from build123d import *

# Parameters (mm, degrees)
BOSS_EXTRUDE1_DEPTH      = 8.5
CUT_EXTRUDE4_DEPTH       = 12
FILLET1_R                = 3
CUT_EXTRUDE5_DEPTH       = 46.354741112
CUT_EXTRUDE5_DEPTH_BACK  = 46.354741112
SKETCH6_W                = 4.541260622
SKETCH6_H                = 2
CUT_EXTRUDE6_START       = 1
CUT_EXTRUDE6_DEPTH       = 3
CUT_EXTRUDE7_REACH       = 47.355
CUT_EXTRUDE7_END_RADIUS  = 42.2
SKETCH8_W                = 25
SKETCH8_H                = 3
BOSS_EXTRUDE2_START      = 6.5
BOSS_EXTRUDE2_DEPTH      = 3
FILLET2_R                = 5
SKETCH10_R               = 11
CUT_EXTRUDE8_DEPTH       = 2
CUT_EXTRUDE9_REACH       = 63.124
SKETCH11_R               = 3.75
FILLET3_R                = 7.5
CUT_EXTRUDE10_DEPTH      = 61.534679882
CUT_EXTRUDE10_DEPTH_BACK = 61.534679882
SKETCH12_W               = 19.340558592
SKETCH12_H               = 3


# Read off the part's stored shape, not the designer's step: Cut-Extrude6
with BuildPart() as part:
    # Sketch1 → Boss-Extrude1 (new, symmetric)
    with BuildSketch(Plane(origin=(0, 0, 0), x_dir=(1, 0, 0), z_dir=(0, 1, 0))):
        with BuildLine():
            Line((-39.278701549, 15), (39.278701549, 15))
            ThreePointArc((39.278701549, 15), (41.95, 0), (39.278701549, -15))
            Line((39.278701549, -15), (-39.278701549, -15))
            ThreePointArc((-39.278701549, -15), (-41.95, 0), (-39.278701549, 15))
        make_face()
    extrude(amount=BOSS_EXTRUDE1_DEPTH, both=True)

    # Sketch5 → Cut-Extrude4 (cut)
    with BuildSketch(Plane(origin=(0, 8.5, 0), x_dir=(1, 0, 0), z_dir=(0, 1, 0))):
        with BuildLine():
            Line((-37.408739378, 15), (34.445827296, 15))
            ThreePointArc((34.445827296, 15), (37.45, 0), (34.445827296, -15))
            Line((34.445827296, -15), (-37.408739378, -15))
            ThreePointArc((-37.408739378, -15), (-40.2, 0), (-37.408739378, 15))
        make_face()
    extrude(amount=-CUT_EXTRUDE4_DEPTH, mode=Mode.SUBTRACT)

    # Fillet1
    fillet1_edges = [part.edges().sort_by_distance(p)[0] for p in [
        (-40.2, -3.5, 0),
        (37.45, -3.5, 0),
        (-41.95, -8.5, 0),
        (41.95, -8.5, 0),
    ]]
    fillet(fillet1_edges, radius=FILLET1_R)

    # Sketch6 → Cut-Extrude5 (cut, two sides: drawn at the far end of the back side and taken through both)
    with BuildSketch(Plane.XY.offset(-CUT_EXTRUDE5_DEPTH_BACK)):
        with Locations((-39.679369689, 7.5)):
            Rectangle(SKETCH6_W, SKETCH6_H)
    extrude(amount=CUT_EXTRUDE5_DEPTH + CUT_EXTRUDE5_DEPTH_BACK, mode=Mode.SUBTRACT)

    # Cut-Extrude6 outline → Cut-Extrude6 (cut)
    with BuildSketch(Plane(origin=(0, 0, 0), x_dir=(1, 0, 0), z_dir=(0, 1, 0)).offset(CUT_EXTRUDE6_START)):
        with BuildLine():
            ThreePointArc((-40.987968885, -4.25), (-40.485797555, -7.777069093), (-39.691352248, -11.25))
            Line((-39.691352248, -11.25), (-38.653798077, -11.25))
            ThreePointArc((-38.653798077, -11.25), (-39.468108328, -7.778438147), (-39.982857905, -4.25))
            Line((-39.982857905, -4.25), (-40.987968885, -4.25))
        make_face()
        with BuildLine():
            Line((-40.987968885, 4.25), (-39.982857905, 4.25))
            ThreePointArc((-39.982857905, 4.25), (-39.468108328, 7.778438147), (-38.653798077, 11.25))
            Line((-38.653798077, 11.25), (-39.691352248, 11.25))
            ThreePointArc((-39.691352248, 11.25), (-40.485797555, 7.777069093), (-40.987968885, 4.25))
        make_face()
    extrude(amount=CUT_EXTRUDE6_DEPTH, mode=Mode.SUBTRACT)

    # Cut-Extrude7: up to this cylinder (the profile starts inside it)
    cut_extrude7_end = Plane(origin=(-1.5, 0.5, 0), z_dir=(0, -1, 0)) * Cylinder(CUT_EXTRUDE7_END_RADIUS, 180.11, mode=Mode.PRIVATE)
    # Sketch8 → Cut-Extrude7 (cut, up to the surface)
    with BuildSketch(Plane(origin=(0, 0, 0), x_dir=(0, 0, -1), z_dir=(1, 0, 0)), mode=Mode.PRIVATE) as cut_extrude7_sk1:
        with Locations((0, 0.5)):
            Rectangle(SKETCH8_W, SKETCH8_H)
    cut_extrude7_tool1 = extrude(cut_extrude7_sk1.sketch, amount=CUT_EXTRUDE7_REACH, mode=Mode.PRIVATE) & cut_extrude7_end
    add(cut_extrude7_tool1.solids().sort_by_distance((0, 0.5, 0))[0], mode=Mode.SUBTRACT)

    # Sketch9 → Boss-Extrude2 (add)
    with BuildSketch(Plane(origin=(0, 0, 0), x_dir=(1, 0, 0), z_dir=(0, 1, 0)).offset(BOSS_EXTRUDE2_START)):
        with BuildLine():
            Line((-53.356504155, 20.178365938), (-39.278701549, 15))
            ThreePointArc((-39.278701549, 15), (-41.95, 0), (-39.278701549, -15))
            Line((-39.278701549, -15), (-53.356504155, -20.178365938))
            ThreePointArc((-53.356504155, -20.178365938), (-56.95, 0), (-53.356504155, 20.178365938))
        make_face()
    extrude(amount=-BOSS_EXTRUDE2_DEPTH)

    # Fillet2
    fillet2_edges = [part.edges().sort_by_distance(p)[0] for p in [
        (-53.356504155, 5, 20.178365938),
        (-53.356504155, 5, -20.178365938),
    ]]
    fillet(fillet2_edges, radius=FILLET2_R)

    # Sketch10 → Cut-Extrude8 (cut)
    with BuildSketch(Plane(origin=(0, -3.5, 0), x_dir=(1, 0, 0), z_dir=(0, 1, 0))):
        with Locations(Location((0, 0, 0), (0, 0, 270))):
            Circle(SKETCH10_R)
    extrude(amount=-CUT_EXTRUDE8_DEPTH, mode=Mode.SUBTRACT)

    # Sketch11 → Cut-Extrude9 (cut, up to next)
    with BuildSketch(Plane(origin=(0, -3.5, 0), x_dir=(1, 0, 0), z_dir=(0, 1, 0)), mode=Mode.PRIVATE) as cut_extrude9_sk1:
        with Locations(Location((0, 0, 0), (0, 0, 270))):
            Circle(SKETCH11_R)
    cut_extrude9_tool1 = extrude(cut_extrude9_sk1.sketch, amount=-CUT_EXTRUDE9_REACH, mode=Mode.PRIVATE) & part.part
    add(cut_extrude9_tool1.solids().sort_by_distance((0, -3.5, 0))[0], mode=Mode.SUBTRACT)

    # Fillet3
    fillet3_edges = [part.edges().sort_by_distance(p)[0] for p in [
        (-41.95, 3.5, 0),
    ]]
    fillet(fillet3_edges, radius=FILLET3_R)

    # Sketch12 → Cut-Extrude10 (cut, two sides: drawn at the far end of the back side and taken through both)
    with BuildSketch(Plane.XY.offset(-CUT_EXTRUDE10_DEPTH_BACK)):
        with Locations((38.128696485, 7)):
            Rectangle(SKETCH12_W, SKETCH12_H)
    extrude(amount=CUT_EXTRUDE10_DEPTH + CUT_EXTRUDE10_DEPTH_BACK, mode=Mode.SUBTRACT)


solid = part.part
Read the model definition and answer for the solid it produces. Units are mm, in the model's axes. A direction names the side the tool comes from. Round coordinates to 2 decimals unless told otherwise and drop trailing zeros. Write each loop counter-clockwise with the first axis right and the second up, starting at its lowest first coordinate (ties: lowest second). Pieces come first, ordered by that corner, then holes.
1. The part is cut by section A-A, the plane x = 0. Determine the outline of the cut face in (y, z), then the cut area to 3 significant figures.
2. The part is cut by section D-D, the plane x = 22. Determine the outline of the cut face in (y, z).
3. Straight lines are drawn through the part: L1, parallel to X at y = -4.55, z = 0; L2, parallel to Y at x = -3, z = 11.5; L3, parallel to Z at x = -22, y = -6.5. For each, find the intervals that lie inside material, in ascending order.
4. Given pin 1 Ø6 at (x, y) = (31, -2) entering from -Z; pin 2 Ø1.2 at (x, z) = (-39.5, -7) entering from -Y; pin 3 Ø1.6 at (x, z) = (38, 0.5) entering from +Y, each flat-ended and moving along its own axis, determine where each tip first touches the part or whether it passes through.
5. Which of the six approach directions +Z, -Z, +X, -X, +Y, -Y give full straight-line access (tool end or side, diameter ignored) to faces 1 (the face through (39, 5.5, 0)), 2 (the face through (37.45, 3.21, -0.22)), 3 (the face through (37, 0, 12.5))?
6. The part is cut by section C-C, the plane y = -6.75. Determine the outline of the cut face in (x, z).
7. The part is cut by section B-B, the plane z = 0. Determine the outline of the cut face in (x, y).
8. Determine the mould class of faces 4 (the face through (-42.78, 3.66, 16.29)), 5 (the face through (-40, 1, 8)), 6 (the face through (-41.95, -4.74, 0.21)) for opening direction Z: pulls with the +Z half, pulls with the -Z half, needs draft (parallel to the pull), parting line crosses it, or undercut.
Values:
1. outline: (-8.5, -15) - (-3.5, -15) - (-3.5, -11) - (-5.5, -11) - (-5.5, -3.75) - (-8.5, -3.75) - close; (-8.5, 3.75) - (-5.5, 3.75) - (-5.5, 11) - (-3.5, 11) - (-3.5, 15) - (-8.5, 15) - close
1. area: 83.5 mm2
2. outline: (-8.5, -15) - (-3.5, -15) - (-3.5, 15) - (-8.5, 15) - close
3. L1: x = -41.95 to -11, 11 to 41.95
3. L2: y = -8.5 to -3.5
3. L3: z = -15 to 15
4. pin 1: stops at z = -15
4. pin 2: stops at y = -8.45
4. pin 3: stops at y = 5.5
5. face 1: +Z, -Z, +X, +Y
5. face 2: +Y
5. face 3: none
6. outline: (-38.99, -15) - (38.99, -15) arc R43.18 ccw to (38.99, 15) - (-38.99, 15) arc R43.18 ccw to start; hole circle Ø7.5 at (0, 0)
7. outline: (-56.95, 3.5) - (-49.45, 3.5) arc R7.5 cw to (-41.95, -4) - (-41.95, -5.5) arc R3 ccw to (-38.95, -8.5) - (-3.75, -8.5) - (-3.75, -5.5) - (-11, -5.5) - (-11, -3.5) - (-37.2, -3.5) arc R3 cw to (-40.2, -0.5) - (-40.2, 6.5) - (-56.95, 6.5) - close; (3.75, -8.5) - (38.95, -8.5) arc R3 ccw to (41.95, -5.5) - (41.95, 5.5) - (37.45, 5.5) - (37.45, 2) - (40.7, 2) - (40.7, -1) - (37.41, -1) arc R3 cw to (34.45, -3.5) - (11, -3.5) - (11, -5.5) - (3.75, -5.5) - close
8. face 4: pulls with the +Z half
8. face 5: undercut
8. face 6: parting line crosses it
